Verification items for the finished model (mm, model axes). A direction names the side the tool comes from. Give positions to 0.01 mm unless a question says otherwise; leave off trailing zeros. Order: outer loops, then holes, each group sorted by start corner. A loop starts at its lowest first (then second) coordinate and runs counter-clockwise, first axis right, second up. Notation, with made-up numbers: (27, 33.5) -> (75, 33.5) arc R24 cw to (75, 52.5) -> close; hole circle Ø4 at (-5.75, 89). An arc over 180 degrees is marked (long way). One line per question, with ' | ' between items. Start each with the question number.
Q1. Section check A-A on x = 0. Record the cut outline in (y, z).
Q2. Go/stop test with flat-tipped pins: pin 1 (10 mm diameter, centred on x = 17, y = 2, fed in from -Z); pin 2 (2 mm diameter, centred on x = 11, y = -1.5, fed in from +Z). Record where each tip stops, or that it passes through.
Q3. Material ranges on probe 1 along Y at (x, z) = (0, 2.3); probe 2 along Z at (x, y) = (13.5, -6.5); probe 3 along Y at (x, z) = (0, 0.4), recorded low to high. Write a range as [from, to].
Q4. Access from +Z, -Z, +X, -X, +Y, -Y to the whole of each face (thin tool, end or side, straight path). Record for faces 1 (the flat face through (1, 3, 3.4)), 2 (the flat face through (0, 6, 2)).
from build123d import *

# Parameters (mm, degrees)
SKETCH_R        = 25
PAD_DEPTH       = 2
SKETCH001_R     = 3
POCKET_DEPTH    = 5
SKETCH002_R     = 5
PAD001_DEPTH    = 1.4
PAD001_FACE6_R  = 3
POCKET001_DEPTH = 5
FILLET_R        = 1
CHAMFER_SIZE    = 1


with BuildPart() as part:
    # Sketch → Pad (new body)
    with BuildSketch(Plane.XY):
        Circle(SKETCH_R)
    extrude(amount=PAD_DEPTH)

    # Sketch001 (on Face3 of Pad) → Pocket (cut)
    with BuildSketch(Plane.XY.offset(2)):
        Circle(SKETCH001_R)
    extrude(amount=-POCKET_DEPTH, mode=Mode.SUBTRACT)

    # Sketch002 (on Face3 of Pocket) → Pad001 (join)
    with BuildSketch(Plane.XY.offset(2)):
        Circle(SKETCH002_R)
    extrude(amount=PAD001_DEPTH)

    # Pad001 Face6 → Pocket001 (cut)
    with BuildSketch(Plane(origin=(0, 0, 2), x_dir=(0, -1, 0), z_dir=(0, 0, -1))):
        Circle(PAD001_FACE6_R)
    extrude(amount=-POCKET001_DEPTH, mode=Mode.SUBTRACT)

    # Fillet
    fillet_edges = [part.edges().sort_by_distance(p)[0] for p in [
        (-25, 0, 2),
    ]]
    fillet(fillet_edges, radius=FILLET_R)

    # Chamfer
    chamfer_edges = [part.edges().sort_by_distance(p)[0] for p in [
        (-5, 0, 3.4),
    ]]
    chamfer(chamfer_edges, length=CHAMFER_SIZE)


solid = part.part
Filled in:
1) outline: (-25, 0) -> (-3, 0) -> (-3, 3.4) -> (-4, 3.4) -> (-5, 2.4) -> (-5, 2) -> (-24, 2) arc R1 ccw to (-25, 1) -> close; (3, 0) -> (25, 0) -> (25, 1) arc R1 ccw to (24, 2) -> (5, 2) -> (5, 2.4) -> (4, 3.4) -> (3, 3.4) -> close
2) pin 1: z = 0 | pin 2: z = 2
3) probe 1: [-5, -3], [3, 5] | probe 2: [0, 2] | probe 3: [-25, -3], [3, 25]
4) face 1: +Z, +X, -X, +Y, -Y | face 2: +Z
